Autodesk Inventor part; units mm, degrees
ref_plane "YZ Plane" through (0, 0, 0) normal (1, 0, 0) x (0, 1, 0)
ref_plane "XZ Plane" through (0, 0, 0) normal (0, 1, 0) x (-1, 0, 0)
ref_plane "XY Plane" through (0, 0, 0) normal (0, 0, 1) x (1, 0, 0)
sketch "Sketch1" plane through (0, 0, 0) normal (0, 1, 0) x (-1, 0, 0)
  line L0 (0, 0) -> (30, 0)
  line L1 (30, 0) -> (30, -30)
  line L2 (30, -30) -> (0, -30)
  line L3 (0, -30) -> (0, 0)
  dimension "d0" = 30
  dimension "d1" = 30
extrude "Extrusion1" add sketch "Sketch1" along normal blind 2
ref_plane "Work Plane1" through (-13, 0, 0) normal (1, 0, 0) x (0, 0, -1)
sketch "Sketch2" plane through (-13, 0, 0) normal (1, 0, 0) x (0, 0, -1)
  line L0 (30, 2) -> (0, 2)
  line L1 (19, 2) -> (16.1597, 10.8569)
  line L2 (11, 2) -> (13.6568, 10.8341)
  arc A0 (16.1597, 10.8569) -> (13.6568, 10.8341) centre (14.9118, 10.4567) ccw
  line L3 (0, 0) -> (0, 2)
  dimension "d5" = 11
  dimension "d6" = 8
extrude "Extrusion2" add sketch "Sketch2" against normal blind 4
properties part number "servo-mount"
Verification items for the finished model (mm, model axes). A direction names the side the tool comes from. Give positions to 0.01 mm unless a question says otherwise; leave off trailing zeros. Write each loop counter-clockwise with the first axis right and the second up, starting at its lowest first coordinate (ties: lowest second). Pieces come first, ordered by that corner, then holes.
(1) Cross-section at D-D (z = -15.5). Enter the section's corners in (x, y).
(2) Access from +Z, -Z, +X, -X, +Y, -Y to the whole of each face (thin tool, end or side, straight path). Record for faces 1 (the face through (-17, 6, -15)), 2 (the face through (-13, 6, -15)), 3 (the face through (-15, 1, -30)).
(3) Material ranges on line 1 (Y direction, x = -7.25, z = -27); line 2 (X direction, y = 4.75, z = -17); line 3 (Z direction, x = -13.75, y = 4.75), recorded low to high.
(4) Cross-section at C-C (y = 9). Enter the section's corners in (x, z).
(5) Gauge pin test, flat ends, axial feed: pin 1 (1.5 mm diameter, centred on x = -6, z = -21.5, fed in from +Y); pin 2 (4 mm diameter, centred on y = 10.5, z = -15, fed in from +X); pin 3 (6.5 mm diameter, centred on y = 6.5, z = -14, fed in from -X). Record the tip position at first contact, or that the pin passes through.
(6) Cross-section at B-B (z = -27.75). Enter the section's corners in (x, y), plus the area to 3 significant figures.
(7) Cross-section at A-A (x = -14.25). Enter the section's corners in (y, z).
Worked out:
1. outline: (-30, 0) - (0, 0) - (0, 2) - (-13, 2) - (-13, 11.63) - (-17, 11.63) - (-17, 2) - (-30, 2) - close
2. face 1: +Z, -Z, -X, +Y
2. face 2: +Z, -Z, +X, +Y
2. face 3: -Z, +X, -X, +Y, -Y
3. line 1: y = 0 to 2
3. line 2: x = -17 to -13
3. line 3: z = -18.12 to -11.83
4. outline: (-17, -16.76) - (-13, -16.76) - (-13, -13.11) - (-17, -13.11) - close
5. pin 1: stops at y = 2
5. pin 2: stops at x = -13
5. pin 3: stops at x = -17
6. outline: (-30, 0) - (0, 0) - (0, 2) - (-30, 2) - close
6. area: 60.0 mm2
7. outline: (0, -30) - (2, -30) - (2, -19) - (10.86, -16.16) arc R1.31 ccw to (10.83, -13.66) - (2, -11) - (2, 0) - (0, 0) - close
